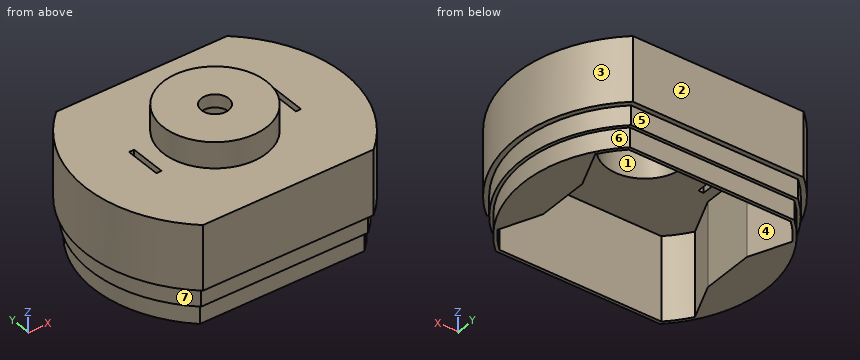
```python
from build123d import *

# Parameters (mm, degrees)
BOSS_EXTRUDE1_DEPTH = 5
SKETCH2_R           = 4
BOSS_EXTRUDE2_DEPTH = 2
BOSS_EXTRUDE3_DEPTH = 1.5
BOSS_EXTRUDE4_DEPTH = 1.5
SKETCH5_W           = 12.75
SKETCH5_H           = 4
CUT_EXTRUDE1_DEPTH  = 6.5
SKETCH6_R           = 3
CUT_EXTRUDE2_DEPTH  = 2.5
SKETCH7_R           = 1.05
CUT_EXTRUDE3_DEPTH  = 2.5
SKETCH8_W           = 0.4
SKETCH8_H           = 2.8
CUT_EXTRUDE4_DEPTH  = 2.5


with BuildPart() as part:
    # Sketch1 → Boss-Extrude1 (new body)
    with BuildSketch(Plane.XY):
        with BuildLine():
            Line((-6.615, 7.5), (6.615, 7.5))
            ThreePointArc((6.615, 7.5), (10.000621722, 0), (6.615, -7.5))
            Line((6.615, -7.5), (-6.615, -7.5))
            ThreePointArc((-6.615, -7.5), (-10.000621722, 0), (-6.615, 7.5))
        make_face()
    extrude(amount=BOSS_EXTRUDE1_DEPTH)

    # Sketch2 → Boss-Extrude2 (add)
    with BuildSketch(Plane.XY.offset(5)):
        Circle(SKETCH2_R)
    extrude(amount=BOSS_EXTRUDE2_DEPTH)

    # Sketch3 → Boss-Extrude3 (add)
    with BuildSketch(Plane(origin=(0, 0, 0), x_dir=(-1, 0, 0), z_dir=(0, 0, -1))):
        with BuildLine():
            Line((-6.469779318, -7.12), (6.469779318, -7.12))
            ThreePointArc((6.469779318, -7.12), (9.620621722, 0), (6.469779318, 7.12))
            Line((6.469779318, 7.12), (-6.469779318, 7.12))
            ThreePointArc((-6.469779318, 7.12), (-9.620621722, 0), (-6.469779318, -7.12))
        make_face()
    extrude(amount=BOSS_EXTRUDE3_DEPTH)

    # Sketch4 → Boss-Extrude4 (add)
    with BuildSketch(Plane(origin=(0, 0, -1.5), x_dir=(-1, 0, 0), z_dir=(0, 0, -1))):
        with BuildLine():
            Line((-6.372434651, -6.87), (6.372434651, -6.87))
            ThreePointArc((6.372434651, -6.87), (9.370621722, 0), (6.372434651, 6.87))
            Line((6.372434651, 6.87), (-6.372434651, 6.87))
            ThreePointArc((-6.372434651, 6.87), (-9.370621722, 0), (-6.372434651, -6.87))
        make_face()
    extrude(amount=BOSS_EXTRUDE4_DEPTH)

    # Sketch5 → Cut-Extrude1 (cut)
    with BuildSketch(Plane(origin=(0, 0, -3), x_dir=(-1, 0, 0), z_dir=(0, 0, -1))):
        with BuildLine():
            Line((-6.374378278, -2), (-7.630621722, -4.995748192))
            ThreePointArc((-7.630621722, -4.995748192), (-6.9993793, -5.847374828), (-6.273579557, -6.62))
            Line((-6.273579557, -6.62), (6.273579557, -6.62))
            ThreePointArc((6.273579557, -6.62), (7.004508128, -5.841230625), (7.639378278, -4.982348672))
            Line((7.639378278, -4.982348672), (6.375621722, -2))
            Line((6.375621722, -2), (-6.374378278, -2))
        make_face()
        with Locations((0.000621722, 0)):
            Rectangle(SKETCH5_W, SKETCH5_H)
        with BuildLine():
            Line((6.375621722, 2), (7.639378278, 4.982348672))
            ThreePointArc((7.639378278, 4.982348672), (7.004508128, 5.841230625), (6.273579557, 6.62))
            Line((6.273579557, 6.62), (-6.273579557, 6.62))
            ThreePointArc((-6.273579557, 6.62), (-6.9993793, 5.847374828), (-7.630621722, 4.995748192))
            Line((-7.630621722, 4.995748192), (-6.374378278, 2))
            Line((-6.374378278, 2), (6.375621722, 2))
        make_face()
    extrude(amount=-CUT_EXTRUDE1_DEPTH, mode=Mode.SUBTRACT)

    # Sketch6 → Cut-Extrude2 (cut)
    with BuildSketch(Plane(origin=(0, 0, 3.5), x_dir=(-1, 0, 0), z_dir=(0, 0, -1))):
        Circle(SKETCH6_R)
    extrude(amount=-CUT_EXTRUDE2_DEPTH, mode=Mode.SUBTRACT)

    # Sketch7 → Cut-Extrude3 (cut)
    with BuildSketch(Plane(origin=(0, 0, 6), x_dir=(-1, 0, 0), z_dir=(0, 0, -1))):
        Circle(SKETCH7_R)
    extrude(amount=-CUT_EXTRUDE3_DEPTH, mode=Mode.SUBTRACT)

    # Sketch8 → Cut-Extrude4 (cut)
    with BuildSketch(Plane(origin=(0, 0, 3.5), x_dir=(-1, 0, 0), z_dir=(0, 0, -1))):
        with Locations((-5.4, 0)):
            Rectangle(SKETCH8_W, SKETCH8_H)
        with Locations((5.4, 0)):
            Rectangle(SKETCH8_W, SKETCH8_H)
    extrude(amount=-CUT_EXTRUDE4_DEPTH, mode=Mode.SUBTRACT)


solid = part.part
```
Check sheet for the modelled part. Datum: model origin and axes. Units: mm. Face numbers are marked on the shaded views. A direction names the side the tool comes from. Round coordinates to 2 decimals unless told otherwise and drop trailing zeros. Loops run counter-clockwise (first coordinate to the right, second up) from the corner with the lowest first, then second, coordinate; pieces in that order, holes last. Notation, with made-up numbers: (34.5, -5) -> (38.5, -5) arc R28 cw to (38.5, 28) -> close; hole circle Ø7 at (-11, 48.25). An arc over 180 degrees is marked (long way). Write item = value, one per line. Start each with the question number.
1) Sectioned sample at C-C, the plane z = 4.25. Record the cut outline in (x, y) (3 decimals).
2) Set-up check for the marked faces 4, 5, 6 and 7: record each of +Z, -Z, +X, -X, +Y, -Y from which the full face is reachable in a straight line by a thin tool's end or side.
3) Gauge pin test, flat ends, axial feed: pin 1 Ø1.2 at (x, z) = (1.5, -2) entering from -Y; pin 2 Ø7 at (x, y) = (0, 0) entering from -Z; pin 3 Ø1 at (y, z) = (5, 3) entering from -X. Record the tip position at first contact, or that the pin passes through.
4) Thickness scan on probe 1 along Y at (x, z) = (0, 6.5); probe 2 along Y at (x, z) = (3.25, -2.5); probe 3 along Z at (x, y) = (-1.5, -4.25). Record the ranges inside material, lowest first.
5) Sectioned sample at D-D, the plane y = 3.5. Record the cut outline in (x, z).
6) Sectioned sample at B-B, the plane x = 6. Record the cut outline in (y, z), plus the area to 3 significant figures.
7) Sectioned sample at A-A, the plane x = 0. Record the cut outline in (y, z), plus the area to 3 significant figures.
8) Release check for a two-part mould opening along Y. For the marked faces 1, 2 and 3 record: released by +Y, released by -Y, zero draft, split by the parting line, or undercut.
Results are:
q1.outline = (-6.615, -7.5) -> (6.615, -7.5) arc R10 ccw to (6.615, 7.5) -> (-6.615, 7.5) arc R10 ccw to start; hole (-5.6, -1.4) -> (-5.2, -1.4) -> (-5.2, 1.4) -> (-5.6, 1.4) -> close; hole circle Ø6 at (0, 0); hole (5.2, -1.4) -> (5.6, -1.4) -> (5.6, 1.4) -> (5.2, 1.4) -> close
q2.face_4 = -Z
q2.face_5 = -Z, +X, -X, +Y
q2.face_6 = -Z, +X
q2.face_7 = -Z, -X
q3.pin_1 = -7.12
q3.pin_2 = 3.5
q3.pin_3 = -8.93
q4.probe_1 = -4 to -1.05, 1.05 to 4
q4.probe_2 = -6.87 to -6.62, 6.62 to 6.87
q4.probe_3 = 3.5 to 5
q5.outline = (-9.37, 0) -> (-8.96, 0) -> (-8.96, -1.5) -> (-8.69, -1.5) -> (-8.69, -3) -> (-7.01, -3) -> (-7.01, 3.5) -> (7, 3.5) -> (7, -3) -> (8.69, -3) -> (8.69, -1.5) -> (8.96, -1.5) -> (8.96, 0) -> (9.37, 0) -> (9.37, 5) -> (1.94, 5) -> (1.94, 7) -> (-1.94, 7) -> (-1.94, 5) -> (-9.37, 5) -> close
q6.outline = (-7.5, 0) -> (-7.12, 0) -> (-7.12, -1.5) -> (-6.87, -1.5) -> (-6.87, -3) -> (-6.62, -3) -> (-6.62, 3.5) -> (6.62, 3.5) -> (6.62, -3) -> (6.87, -3) -> (6.87, -1.5) -> (7.12, -1.5) -> (7.12, 0) -> (7.5, 0) -> (7.5, 5) -> (-7.5, 5) -> close
q6.area = 30.9 mm^2
q7.outline = (-7.5, 0) -> (-7.12, 0) -> (-7.12, -1.5) -> (-6.87, -1.5) -> (-6.87, -3) -> (-6.62, -3) -> (-6.62, 3.5) -> (-3, 3.5) -> (-3, 6) -> (-1.05, 6) -> (-1.05, 7) -> (-4, 7) -> (-4, 5) -> (-7.5, 5) -> close; (1.05, 6) -> (3, 6) -> (3, 3.5) -> (6.62, 3.5) -> (6.62, -3) -> (6.87, -3) -> (6.87, -1.5) -> (7.12, -1.5) -> (7.12, 0) -> (7.5, 0) -> (7.5, 5) -> (4, 5) -> (4, 7) -> (1.05, 7) -> close
q7.area = 29.8 mm^2
q8.face_1 = undercut
q8.face_2 = released by +Y
q8.face_3 = split by the parting line
